Could you check a few things on this drawing? It's one solid part, dimensions in mm from its lowest x, y, z. Give positions to 0.01 mm unless a question says otherwise; leave off trailing zeros. Write each loop counter-clockwise with the first axis right and the second up, starting at its lowest first coordinate (ties: lowest second). Pieces come first, ordered by that corner, then holes. Notation, with made-up numbers: (28, -8) -> (32, -8) arc R27 ccw to (32, 13) -> close; hole circle Ø9 at (41.25, -35). An arc over 180 degrees is marked (long way). Answer as CSV lines item,"result". Start each with the question number.
1. I need wall thicknesses on line 1 (Y direction, x = 35, z = 4.7); line 2 (Y direction, x = 8, z = 2.1); line 3 (X direction, y = 34.5, z = 0.65) (1 decimal). Which ranges of each line are inside material? Lowest first, please. Write a range as [from, to].
2. If we mould it in two halves opening along X, with no side actions, what happens to the marked faces 1, 2 and 3? For each: pulls with the +X half, pulls with the -X half, needs draft (parallel to the pull), parting line crosses it, or undercut.
3. If we section it at B-B on y = 15.5: Write out the boundary of the cut face in (x, z) (1 decimal).
4. If we section it at A-A on x = 35: Write out the boundary of the cut face in (y, z), plus the area to 3 significant figures.
5. If we section it at D-D on x = 53: Write out the boundary of the cut face in (y, z), plus the area to 3 significant figures.
6. I'm going to push flat-ended pins straight in: P1, Ø1.9, axis at x = 60.98, y = 50, coming from the +Z side; P2, Ø3.5, axis at x = 60.98, y = 20, coming from the -Z side; P3, Ø1, axis at x = 41.5, z = 4, coming from the +Y side; P4, Ø1.5, axis at x = 35, z = 3.5, coming from the -Y side. Where does each tip first touch, or does it pass through?
7. If we section it at C-C on z = 2.45: Write out the boundary of the cut face in (x, y).
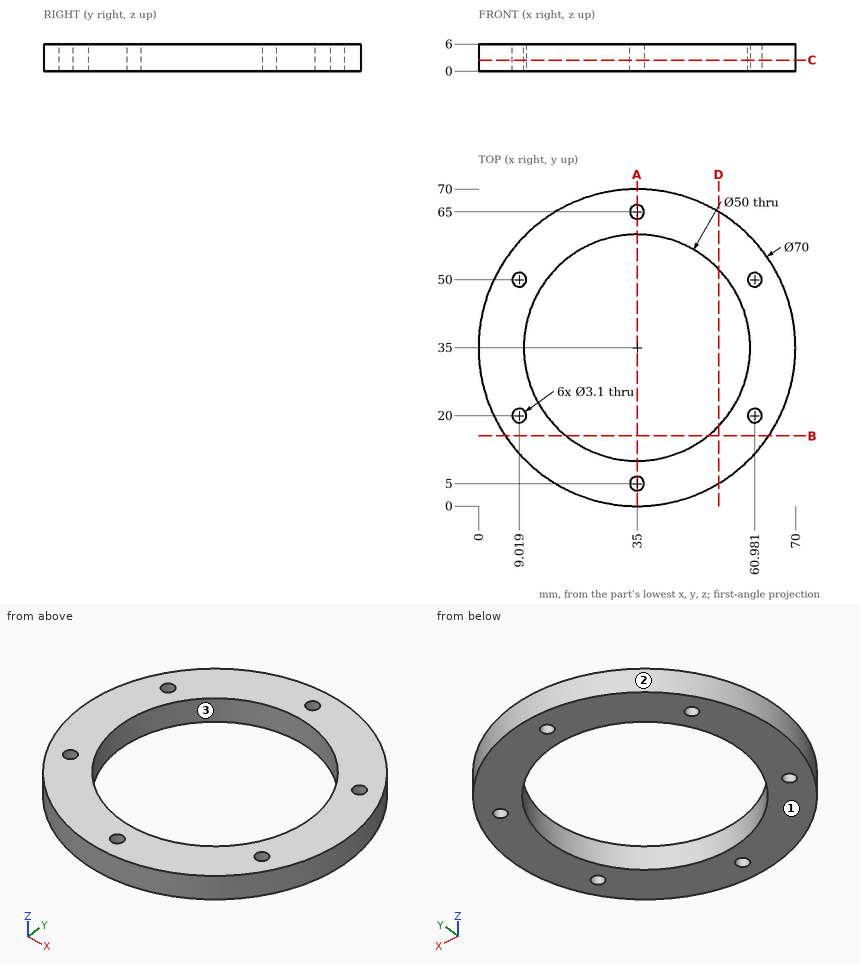
Computed values:
1,line 1,"y = [0, 3.45], [6.55, 10], [60, 63.45], [66.55, 70]"
1,line 2,"y = [12.73, 18.83], [21.17, 48.83], [51.17, 57.27]"
1,line 3,"x = [0, 10], [60, 70]"
2,face 1,"needs draft"
2,face 2,"parting line crosses it"
2,face 3,"undercut"
3,outline,"(5.9, 0) -> (19.4, 0) -> (19.4, 6) -> (5.9, 6) -> close; (50.6, 0) -> (64.1, 0) -> (64.1, 6) -> (50.6, 6) -> close"
4,outline,"(0, 0) -> (3.45, 0) -> (3.45, 6) -> (0, 6) -> close; (6.55, 0) -> (10, 0) -> (10, 6) -> (6.55, 6) -> close; (60, 0) -> (63.45, 0) -> (63.45, 6) -> (60, 6) -> close; (66.55, 0) -> (70, 0) -> (70, 6) -> (66.55, 6) -> close"
4,area,"82.8 mm2"
5,outline,"(4.98, 0) -> (17.65, 0) -> (17.65, 6) -> (4.98, 6) -> close; (52.35, 0) -> (65.02, 0) -> (65.02, 6) -> (52.35, 6) -> close"
5,area,"152 mm2"
6,P1,"passes through"
6,P2,"stops at z = 0"
6,P3,"stops at y = 69.48"
6,P4,"stops at y = 0"
7,outline,"circle Ø70 at (35, 35); hole circle Ø3.1 at (9.02, 20); hole circle Ø3.1 at (9.02, 50); hole circle Ø50 at (35, 35); hole circle Ø3.1 at (35, 5); hole circle Ø3.1 at (35, 65); hole circle Ø3.1 at (60.98, 20); hole circle Ø3.1 at (60.98, 50)"
